from build123d import *

# Parameters (mm, degrees)
F0_W     = 300
F0_H     = 100
F1_DEPTH = 30
F3_DEPTH = 20
F4_R     = 5
F5_DEPTH = 30.001


with BuildPart() as f1:
    # F0 (on Top) → F1 (new body)
    with BuildSketch(Plane.XY):
        with Locations((150, 50)):
            Rectangle(F0_W, F0_H)
    extrude(amount=F1_DEPTH)

    # F2 (on face) → F3 (cut)
    with BuildSketch(Plane.XY.offset(30)):
        with BuildLine():
            Line((268.83399, 90), (150, 90))
            Line((150, 90), (31.16601, 90))
            ThreePointArc((31.16601, 90), (26.200915, 88.506519), (22.883659, 84.521739))
            ThreePointArc((22.883659, 84.521739), (19.899495, 80.100505), (15.478261, 77.116341))
            ThreePointArc((15.478261, 77.116341), (11.493481, 73.799085), (10, 68.83399))
            Line((10, 68.83399), (10, 50))
            Line((10, 50), (10, 31.16601))
            ThreePointArc((10, 31.16601), (11.493481, 26.200915), (15.478261, 22.883659))
            ThreePointArc((15.478261, 22.883659), (19.899495, 19.899495), (22.883659, 15.478261))
            ThreePointArc((22.883659, 15.478261), (26.200915, 11.493481), (31.16601, 10))
            Line((31.16601, 10), (150, 10))
            Line((150, 10), (268.83399, 10))
            ThreePointArc((268.83399, 10), (273.799085, 11.493481), (277.116341, 15.478261))
            ThreePointArc((277.116341, 15.478261), (280.100505, 19.899495), (284.521739, 22.883659))
            ThreePointArc((284.521739, 22.883659), (288.506519, 26.200915), (290, 31.16601))
            Line((290, 31.16601), (290, 50))
            Line((290, 50), (290, 68.83399))
            ThreePointArc((290, 68.83399), (288.506519, 73.799085), (284.521739, 77.116341))
            ThreePointArc((284.521739, 77.116341), (280.100505, 80.100505), (277.116341, 84.521739))
            ThreePointArc((277.116341, 84.521739), (273.799085, 88.506519), (268.83399, 90))
        make_face()
    extrude(amount=-F3_DEPTH, mode=Mode.SUBTRACT)

    # F4 (on face) → F5 (cut, through all)
    with BuildSketch(Plane.XY.offset(30)):
        with Locations((290, 90)):
            Circle(F4_R)
        with Locations((10, 90)):
            Circle(F4_R)
        with Locations((10, 10)):
            Circle(F4_R)
        with Locations((290, 10)):
            Circle(F4_R)
    extrude(amount=-F5_DEPTH, mode=Mode.SUBTRACT)


solid = f1.part
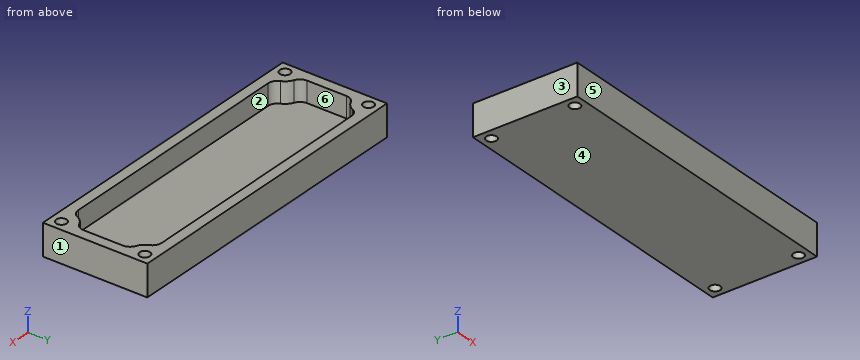
Geometry: final body of the model. Coordinates: model frame, mm. Face numbers are marked on the shaded views. A direction names the side the tool comes from. Round coordinates to 2 decimals unless told otherwise and drop trailing zeros. Order: outer loops, then holes, each group sorted by start corner. A loop starts at its lowest first (then second) coordinate and runs counter-clockwise, first axis right, second up.
Q1. Mould query, pull axis X, two halves, no side actions, for the marked faces 1, 2, 3 and 4. Classes: released by +X, released by -X, zero draft, split by the parting line, or undercut.
Result sheet:
face 1: released by +X
face 2: undercut
face 3: released by -X
face 4: zero draft
Q2. Section C-C, the plane y = 59.5. Output: boundary loops of the cut face in (x, z).
Result sheet:
outline: (0, 0) - (300, 0) - (300, 30) - (290, 30) - (290, 10) - (10, 10) - (10, 30) - (0, 30) - close
Q3. Section A-A, the plane z = 14. Output: boundary loops of the cut face in (x, y).
Result sheet:
outline: (0, 0) - (300, 0) - (300, 100) - (0, 100) - close; hole circle Ø10 at (10, 10); hole circle Ø10 at (10, 90); hole (10, 31.17) arc R9 ccw to (15.48, 22.88) arc R14 cw to (22.88, 15.48) arc R9 ccw to (31.17, 10) - (268.83, 10) arc R9 ccw to (277.12, 15.48) arc R14 cw to (284.52, 22.88) arc R9 ccw to (290, 31.17) - (290, 68.83) arc R9 ccw to (284.52, 77.12) arc R14 cw to (277.12, 84.52) arc R9 ccw to (268.83, 90) - (31.17, 90) arc R9 ccw to (22.88, 84.52) arc R14 cw to (15.48, 77.12) arc R9 ccw to (10, 68.83) - close; hole circle Ø10 at (290, 10); hole circle Ø10 at (290, 90)
Q4. Access query for the marked faces 5 and 6. Directions: +Z, -Z, +X, -X, +Y, -Y. A direction counts if a zero-diameter tool reaches every point of the face in a straight line with its end or side. Return the directions, or none.
Result sheet:
face 5: +Z, -Z, +X, -X, -Y
face 6: +Z
Q5. Pin query (flat end, axial travel): pin 1 (8 mm diameter, centred on x = 290, y = 10, fed in from -Z); pin 2 (24 mm diameter, centred on x = 177.5, y = 40.5, fed in from +Z). Return the tip coordinate at first contact, or that it passes through.
Result sheet:
pin 1: passes through
pin 2: stops at z = 10
Q6. Material intervals for probe 1 along Y at (x, z) = (100, 14.5); probe 2 along Y at (x, z) = (290, 8.25); probe 3 along X at (y, z) = (53, 11.5), sorted ascending.
Result sheet:
probe 1: y = 0 to 10, 90 to 100
probe 2: y = 0 to 5, 15 to 85, 95 to 100
probe 3: x = 0 to 10, 290 to 300
Q7. Section B-B, the plane x = 134. Output: boundary loops of the cut face in (y, z).
Result sheet:
outline: (0, 0) - (100, 0) - (100, 30) - (90, 30) - (90, 10) - (10, 10) - (10, 30) - (0, 30) - close
